Design review of the part shown in the three views and the two pictorial views. Dimensions are in mm from the part's minimum x, y and z. Coordinates: 2 decimals unless noted, no trailing zeros. Order: outer loops, then holes, each group sorted by start corner. A loop starts at its lowest first (then second) coordinate and runs counter-clockwise, first axis right, second up. Notation, with made-up numbers: M 22.5,20 L 26.5,20 A13 cw 26.5,43 Z; hole C 1.5,-22.5 d11. An arc over 180 degrees is marked long. Use CSV: the item, a comma, the result in double quotes.
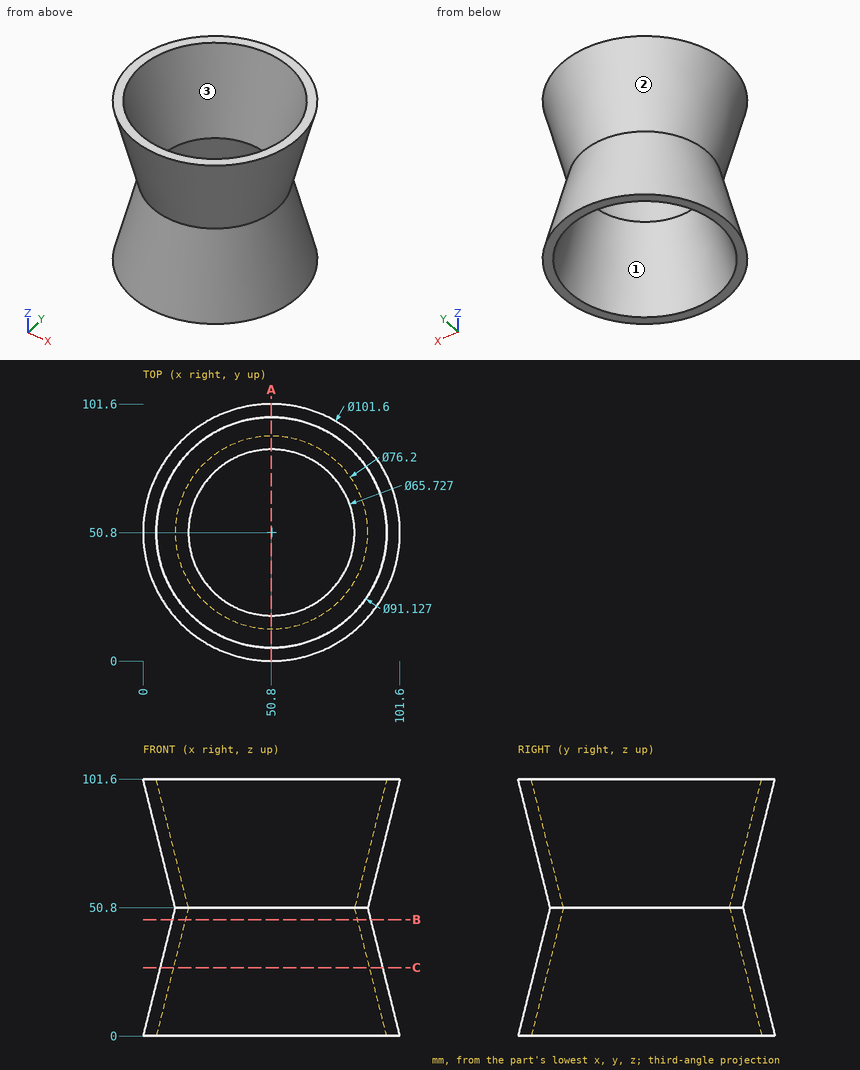
(1) Clearance check with flat-ended pins moving along their axes: P1, Ø8, axis at y = 54, z = 58.5, coming from the +X side (1 decimal); P2, Ø8, axis at x = 82, z = 45, coming from the +Y side (1 decimal); P3, Ø2, axis at y = 48, z = 36.5, coming from the +X side. State where each tip first meets the part, or that it passes through.
The answers:
P1,"stops at x = 91.7"
P2,"stops at y = 79.8"
P3,"stops at x = 92.64"
(2) Add section A-A on x = 50.8. State the section outline as (y, z) points, and give its area (3 significant figures).
The answers:
outline,"M 0,0 L 5.24,0 L 17.94,50.8 L 5.24,101.6 L 0,101.6 L 12.7,50.8 Z; M 83.66,50.8 L 96.36,0 L 101.6,0 L 88.9,50.8 L 101.6,101.6 L 96.36,101.6 Z"
area,"1,060 mm2"
(3) Add section C-C on z = 27. State the section outline as (x, y) points, and give its area (3 significant figures).
The answers:
outline,"C 50.8,50.8 d88.1; hole C 50.8,50.8 d77.63"
area,"1,360 mm2"
(4) Wall thickness on probe 1 along X at (y, z) = (35.5, 59.5) (1 decimal); probe 2 along X at (y, z) = (16, 17) (1 decimal); probe 3 along Y at (x, z) = (37, 63): over which ranges is each line inside the solid? List them lowest first.
The answers:
probe 1,"x = 13.5 to 19.3, 82.3 to 88.1"
probe 2,"x = 19.9 to 28.5, 73.1 to 81.7"
probe 3,"y = 12.03 to 17.64, 83.96 to 89.57"
(5) The part is to be moulded in two halves that separate along Z. For the marked faces 1, 2 and 3, say which applies: pulls with the +Z half, pulls with the -Z half, needs draft (parallel to the pull), parting line crosses it, or undercut.
The answers:
face 1,"pulls with the -Z half"
face 2,"undercut"
face 3,"pulls with the +Z half"
(6) Add section B-B on z = 46. State the section outline as (x, y) points.
The answers:
outline,"C 50.8,50.8 d78.6; hole C 50.8,50.8 d68.13"
